```python
from build123d import *

# Parameters (mm, degrees)
CROQUIS1_W              = 42
CROQUIS1_H              = 32
CROQUIS1_R              = 1.6
SALIENTE_EXTRUIR1_DEPTH = 2
CROQUIS2_W              = 11.5
CROQUIS2_H              = 10
SALIENTE_EXTRUIR2_DEPTH = 12
SALIENTE_EXTRUIR3_START = -1
CROQUIS3_R              = 6.75
SALIENTE_EXTRUIR3_DEPTH = 19.5
CORTAR_EXTRUIR1_START   = -18.5
CROQUIS4_R              = 6.75
CROQUIS4_R_2            = 5.85
CORTAR_EXTRUIR1_DEPTH   = 18.5
CORTAR_EXTRUIR2_START   = -11.5
CROQUIS5_R              = 5.85
CROQUIS5_R_2            = 4.9
CORTAR_EXTRUIR2_DEPTH   = 11.5
SALIENTE_EXTRUIR4_DEPTH = 8


with BuildPart() as part:
    # Croquis1 → Saliente-Extruir1 (new body)
    with BuildSketch(Plane.XY):
        Rectangle(CROQUIS1_W, CROQUIS1_H)
        with Locations((-17.5, 12.25)):
            Circle(CROQUIS1_R, mode=Mode.SUBTRACT)
        with Locations((-17.5, -12.25)):
            Circle(CROQUIS1_R, mode=Mode.SUBTRACT)
        with Locations((17.5, -12.25)):
            Circle(CROQUIS1_R, mode=Mode.SUBTRACT)
        with Locations((17.5, 12.25)):
            Circle(CROQUIS1_R, mode=Mode.SUBTRACT)
    extrude(amount=SALIENTE_EXTRUIR1_DEPTH)

    # Croquis2 → Saliente-Extruir2 (add)
    with BuildSketch(Plane.XY.offset(2)):
        with Locations((15.25, -2)):
            Rectangle(CROQUIS2_W, CROQUIS2_H)
    extrude(amount=SALIENTE_EXTRUIR2_DEPTH)

    # Croquis3 → Saliente-Extruir3 (add)
    with BuildSketch(Plane(origin=(21, 0, 0), x_dir=(0, 0, -1), z_dir=(1, 0, 0)).offset(SALIENTE_EXTRUIR3_START)):
        with Locations(Location((-8.85, -2, 0), (0, 0, 220.27389294))):
            Circle(CROQUIS3_R)
    extrude(amount=SALIENTE_EXTRUIR3_DEPTH)

    # Croquis4 → Cortar-Extruir1 (cut)
    with BuildSketch(Plane(origin=(39.5, 0, 0), x_dir=(0, 0, -1), z_dir=(1, 0, 0)).offset(CORTAR_EXTRUIR1_START)):
        with Locations((-8.85, -2)):
            Circle(CROQUIS4_R)
        with Locations((-8.85, -2)):
            Circle(CROQUIS4_R_2, mode=Mode.SUBTRACT)
    extrude(amount=CORTAR_EXTRUIR1_DEPTH, mode=Mode.SUBTRACT)

    # Croquis5 → Cortar-Extruir2 (cut)
    with BuildSketch(Plane(origin=(39.5, 0, 0), x_dir=(0, 0, -1), z_dir=(1, 0, 0)).offset(CORTAR_EXTRUIR2_START)):
        with Locations((-8.85, -2)):
            Circle(CROQUIS5_R)
        with Locations((-8.85, -2)):
            Circle(CROQUIS5_R_2, mode=Mode.SUBTRACT)
    extrude(amount=CORTAR_EXTRUIR2_DEPTH, mode=Mode.SUBTRACT)

    # Croquis7 → Saliente-Extruir4 (add, symmetric)
    with BuildSketch(Plane(origin=(0, 0, 0), x_dir=(1, 0, 0), z_dir=(0, 1, 0))):
        Polygon((-21, -2), (-21, -5.4), (-35.4, -5.4), (-35.4, -7), (-19.4, -7), (-19.4, -2), align=None)
    extrude(amount=SALIENTE_EXTRUIR4_DEPTH, both=True)


solid = part.part
```
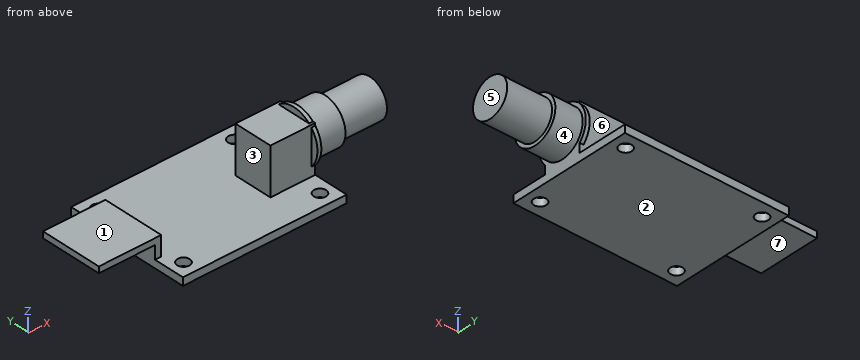
Model file for the job. Use its own axes, mm. Face numbers are marked on the shaded views. A direction names the side the tool comes from. Give positions to 0.01 mm unless a question says otherwise; leave off trailing zeros. Order: outer loops, then holes, each group sorted by start corner. A loop starts at its lowest first (then second) coordinate and runs counter-clockwise, first axis right, second up.
1) Saw through at A-A, the plane x = 17.5. Write the cut outline in (y, z), then the cut area to 3 significant figures.
2) Wall check: probe 1 along Y at (x, z) = (17.5, 0.9); probe 2 along Z at (x, y) = (-21.5, -6.5); probe 3 along Z at (x, y) = (-20, -6). Give the ranges that are in metal, low to high.
3) Pin check, flat tips, straight feed: pin 1 (8 mm diameter, centred on x = 13, y = -0.5, fed in from +Z); pin 2 (5 mm diameter, centred on x = -27.5, y = 2.5, fed in from +Z); pin 3 (9.5 mm diameter, centred on x = -5, y = 2, fed in from +Z); pin 4 (1.9 mm diameter, centred on x = 17.5, y = -12.25, fed in from -Z). Stop position of each tip, or through.
4) Saw through at D-D, the plane x = -17.5. Write the cut outline in (y, z), then the cut area to 3 significant figures.
5) Mould opens along X. For the marked faces 5, 6 and 7 say: +X half, -X half, draft (parallel to the pull), parting line (faces both ways), or undercut.
6) Saw through at C-C, the plane z = 1. Write the cut outline in (x, y).
7) Saw through at B-B, the plane y = 12.25. Write the cut outline in (x, z).
8) 3-axis set-ups, long thin cutter, end or side, ignore diameter. For the marked faces 1, 2, 3 and 4: which of +Z, -Z, +X, -X, +Y, -Y reach the whole face in a straight line?
Computed:
1. outline: (-16, 0) - (-13.85, 0) - (-13.85, 2) - (-16, 2) - close; (-10.65, 0) - (10.65, 0) - (10.65, 2) - (3, 2) - (3, 14) - (-7, 14) - (-7, 2) - (-10.65, 2) - close; (13.85, 0) - (16, 0) - (16, 2) - (13.85, 2) - close
1. area: 171 mm2
2. probe 1: y = -16 to -13.85, -10.65 to 10.65, 13.85 to 16
2. probe 2: z = 5.4 to 7
2. probe 3: z = 0 to 7
3. pin 1: stops at z = 14
3. pin 2: stops at z = 7
3. pin 3: stops at z = 2
3. pin 4: passes through
4. outline: (-16, 0) - (-13.85, 0) - (-13.85, 2) - (-16, 2) - close; (-10.65, 0) - (10.65, 0) - (10.65, 2) - (-10.65, 2) - close; (13.85, 0) - (16, 0) - (16, 2) - (13.85, 2) - close
4. area: 51.2 mm2
5. face 5: +X half
5. face 6: undercut
5. face 7: draft
6. outline: (-21, -16) - (21, -16) - (21, 16) - (-21, 16) - close; hole circle Ø3.2 at (-17.5, -12.25); hole circle Ø3.2 at (-17.5, 12.25); hole circle Ø3.2 at (17.5, -12.25); hole circle Ø3.2 at (17.5, 12.25)
7. outline: (-21, 0) - (-19.1, 0) - (-19.1, 2) - (-21, 2) - close; (-15.9, 0) - (15.9, 0) - (15.9, 2) - (-15.9, 2) - close; (19.1, 0) - (21, 0) - (21, 2) - (19.1, 2) - close
8. face 1: +Z, -X, +Y, -Y
8. face 2: -Z, +X, -X, +Y, -Y
8. face 3: +Z, +Y, -Y
8. face 4: +X
